Design review of the part built by this model. Coordinates are the model's own, in mm. Face numbers are marked on the shaded views. Coordinates: 2 decimals unless noted, no trailing zeros. Write each loop counter-clockwise with the first axis right and the second up, starting at its lowest first coordinate (ties: lowest second). Pieces come first, ordered by that corner, then holes. Notation, with made-up numbers: (82.25, 64.25) - (110.25, 64.25) arc R25 cw to (110.25, 88.25) - close; hole circle Ø1 at (-19.75, -23.5). An arc over 180 degrees is marked (long way). Answer as CSV lines item,"result". Start each with the question number.
Q1. We need section A-A (z = 8.5). Write out the cut boundary in (x, y), plus the area to 3 significant figures.
Q2. We need section C-C (y = -5). Write out the cut boundary in (x, z), plus the area to 3 significant figures.
Q3. We need section B-B (x = 50). Write out the cut boundary in (y, z), plus the area to 3 significant figures.
Q4. Clearance check with flat-ended pins moving along their axes: pin 1 (1.5 mm diameter, centred on x = -41.5, y = -1.5, fed in from -Z); pin 2 (4 mm diameter, centred on x = 30.5, y = -6.5, fed in from -Z); pin 3 (3.5 mm diameter, centred on x = -50, y = 0, fed in from -Z). State where each tip first meets the part, or that it passes through.
Q5. For line 1 along Y through (x, z) = (31.5, 1.75); line 2 along X through (y, z) = (5.25, 8.5); line 3 along X through (y, z) = (8.25, 6.5), list the stretches that pass through material, from the lowest coordinate up. Write a range as [from, to].
Q6. Mouldability with a two-part tool opening along Z and no side actions: class the marked faces 1, 2 and 3 as pulls with the +Z half, pulls with the -Z half, needs draft (parallel to the pull), parting line crosses it, or undercut.
from build123d import *

# Parameters (mm, degrees)
SKETCH_1_W          = 130
SKETCH_1_H          = 24
SKETCH_1_R          = 3
EXTRUDE_1_DEPTH     = 10
SKETCH_2_R          = 4
CUT_EXTRUDE_1_DEPTH = 7


with BuildPart() as part:
    # 草图1 → 凸台-拉伸1 (new body)
    with BuildSketch(Plane.XY):
        Rectangle(SKETCH_1_W, SKETCH_1_H)
        with Locations((-50, 0)):
            Circle(SKETCH_1_R, mode=Mode.SUBTRACT)
        with Locations((50, 0)):
            Circle(SKETCH_1_R, mode=Mode.SUBTRACT)
        Circle(SKETCH_1_R, mode=Mode.SUBTRACT)
        with BuildLine():
            Line((32.5, 6.5), (30.5, 6.5))
            ThreePointArc((30.5, 6.5), (29, 5), (30.5, 3.5))
            Line((30.5, 3.5), (32.5, 3.5))
            ThreePointArc((32.5, 3.5), (34, 5), (32.5, 6.5))
        make_face(mode=Mode.SUBTRACT)
        with BuildLine():
            Line((32.5, -6.5), (30.5, -6.5))
            ThreePointArc((30.5, -6.5), (29, -5), (30.5, -3.5))
            Line((30.5, -3.5), (32.5, -3.5))
            ThreePointArc((32.5, -3.5), (34, -5), (32.5, -6.5))
        make_face(mode=Mode.SUBTRACT)
        with BuildLine():
            Line((-32.5, 6.5), (-30.5, 6.5))
            ThreePointArc((-30.5, 6.5), (-29, 5), (-30.5, 3.5))
            Line((-30.5, 3.5), (-32.5, 3.5))
            ThreePointArc((-32.5, 3.5), (-34, 5), (-32.5, 6.5))
        make_face(mode=Mode.SUBTRACT)
        with BuildLine():
            Line((-32.5, -6.5), (-30.5, -6.5))
            ThreePointArc((-30.5, -6.5), (-29, -5), (-30.5, -3.5))
            Line((-30.5, -3.5), (-32.5, -3.5))
            ThreePointArc((-32.5, -3.5), (-34, -5), (-32.5, -6.5))
        make_face(mode=Mode.SUBTRACT)
    extrude(amount=EXTRUDE_1_DEPTH)

    # 草图2 → 切除-拉伸1 (cut)
    with BuildSketch(Plane(origin=(0, 0, 0), x_dir=(-1, 0, 0), z_dir=(0, 0, -1))):
        with Locations((-31.5, 5)):
            Circle(SKETCH_2_R)
        with Locations((-31.5, -5)):
            Circle(SKETCH_2_R)
        with Locations(Location((31.5, -5, 0), (0, 0, 180))):
            Circle(SKETCH_2_R)
        with Locations(Location((31.5, 5, 0), (0, 0, 180))):
            Circle(SKETCH_2_R)
    extrude(amount=-CUT_EXTRUDE_1_DEPTH, mode=Mode.SUBTRACT)


solid = part.part
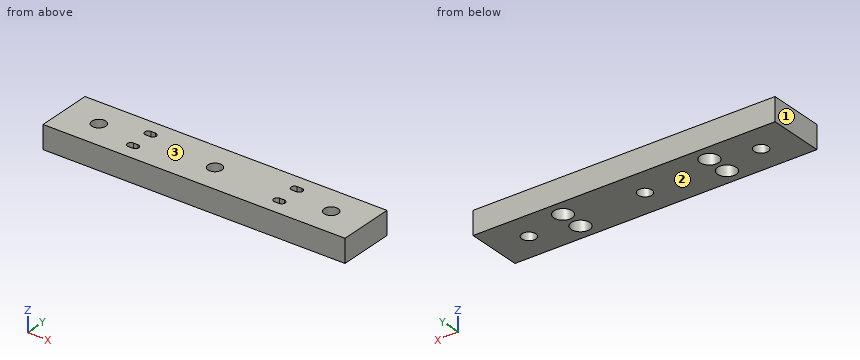
Results list:
1,outline,"(-65, -12) - (65, -12) - (65, 12) - (-65, 12) - close; hole circle Ø6 at (-50, 0); hole (-32.5, -6.5) - (-30.5, -6.5) arc R1.5 ccw to (-30.5, -3.5) - (-32.5, -3.5) arc R1.5 ccw to start; hole (-32.5, 3.5) - (-30.5, 3.5) arc R1.5 ccw to (-30.5, 6.5) - (-32.5, 6.5) arc R1.5 ccw to start; hole circle Ø6 at (0, 0); hole (30.5, -6.5) - (32.5, -6.5) arc R1.5 ccw to (32.5, -3.5) - (30.5, -3.5) arc R1.5 ccw to start; hole (30.5, 3.5) - (32.5, 3.5) arc R1.5 ccw to (32.5, 6.5) - (30.5, 6.5) arc R1.5 ccw to start; hole circle Ø6 at (50, 0)"
1,area,"2,980 mm2"
2,outline,"(-65, 0) - (-35.5, 0) - (-35.5, 7) - (-34, 7) - (-34, 10) - (-65, 10) - close; (-29, 7) - (-27.5, 7) - (-27.5, 0) - (27.5, 0) - (27.5, 7) - (29, 7) - (29, 10) - (-29, 10) - close; (34, 7) - (35.5, 7) - (35.5, 0) - (65, 0) - (65, 10) - (34, 10) - close"
2,area,"1,160 mm2"
3,outline,"(-12, 0) - (-3, 0) - (-3, 10) - (-12, 10) - close; (3, 0) - (12, 0) - (12, 10) - (3, 10) - close"
3,area,"180 mm2"
4,pin 1,"stops at z = 0"
4,pin 2,"stops at z = 7"
4,pin 3,"passes through"
5,line 1,"y = [-12, -9], [-1, 1], [9, 12]"
5,line 2,"x = [-65, -33.98], [-29.02, 29.02], [33.98, 65]"
5,line 3,"x = [-65, -33.83], [-29.17, 29.17], [33.83, 65]"
6,face 1,"needs draft"
6,face 2,"pulls with the -Z half"
6,face 3,"pulls with the +Z half"
